Could you check a few things on this model? Use its own coordinates, in mm. A direction names the side the tool comes from. Give positions to 0.01 mm unless a question says otherwise; leave off trailing zeros. Loops run counter-clockwise (first coordinate to the right, second up) from the corner with the lowest first, then second, coordinate; pieces in that order, holes last. Notation, with made-up numbers: (71.25, 42.25) - (127.25, 42.25) arc R7 cw to (127.25, 48.25) - close; hole circle Ø6 at (22, -21.5). An arc over 180 degrees is marked (long way). Write each question's results on one line, items separated by ' | '. Start each with the question number.
1) I want a section at D-D, the plane y = 44. Write out the boundary of the cut face in (x, z) (3 decimals), and give its area (3 significant figures).
2) I'm going to push flat-ended pins straight in: pin 1 (2 mm diameter, centred on x = 0, z = -22, fed in from +Y); pin 2 (3 mm diameter, centred on x = 0, z = -189, fed in from +Y); pin 3 (1 mm diameter, centred on x = -0.5, y = 2.5, fed in from -Z). Where does each tip first touch, or does it pass through?
3) If we mould it in two halves opening along Y, with no side actions, what happens to faces 1 (the face through (0.044, -31.253, -213.834)), 2 (the face through (0, -21, -216.22)), 3 (the face through (0, -24.244, -107))? For each: +Y half, -Y half, draft (parallel to the pull), parting line (faces both ways), or undercut.
4) I want a section at B-B, the plane x = -1.5. Count the separate pieces of the cut face and the enclosed holes in it, and give its area (3 significant figures).
5) On a 3-axis mill with a long thin cutter (end or side, diameter ignored), from which of +Z, -Z, +X, -X, +Y, -Y can I reach the whole of each face in a straight line? I mean faces 4 (the face through (0, -33.769, -127)), 5 (the face through (0.044, 32.874, -211.617)), 6 (the face through (0.044, 0.201, -216.993)). Say none if no direction works.
6) I want a section at A-A, the plane z = 0. Write out the boundary of the cut face in (x, y) (3 decimals).
7) I want a section at C-C, the plane z = -102.5. Write out the boundary of the cut face in (x, y) (3 decimals).
8) If I drill on probe 1 along Y at (x, z) = (1.25, -196); probe 2 along Y at (x, z) = (0.5, -207); probe 3 along Y at (x, z) = (-0.25, -124.5), over which ranges is the centre line in solid material (lowest first)? Write a range as [from, to].
from build123d import *

# Parameters (mm, degrees)
SKETCH1_R           = 27.5
SKETCH1_R_2         = 3.175
BOSS_EXTRUDE1_DEPTH = 3.175


with BuildPart() as part:
    # Sketch1 → Boss-Extrude1 (new, symmetric)
    with BuildSketch(Plane(origin=(0, 0, 0), x_dir=(0, 0, -1), z_dir=(1, 0, 0))):
        with BuildLine():
            Line((43.290925291, 33.7693), (207.850950123, 33.7693))
            ThreePointArc((207.850950123, 33.7693), (211.66677379, 32.848803409), (214.643231519, 30.28979508))
            ThreePointArc((214.643231519, 30.28979508), (218.030702378, 27.377418378), (222.373445551, 26.329812242))
            Line((222.373445551, 26.329812242), (225.811462365, 26.329812242))
            ThreePointArc((225.811462365, 26.329812242), (234.009351835, 19.645680106), (229.112770692, 10.26983309))
            ThreePointArc((229.112770692, 10.26983309), (224.916562194, 6.758274432), (223.344950123, 1.517163342))
            Line((223.344950123, 1.517163342), (223.344950123, -4.239874171))
            ThreePointArc((223.344950123, -4.239874171), (222.587277992, -7.247924869), (220.495070123, -9.538143699))
            ThreePointArc((220.495070123, -9.538143699), (217.356758318, -12.973471943), (216.220250123, -17.48554799))
            Line((216.220250123, -17.48554799), (216.220250123, -25.4))
            ThreePointArc((216.220250123, -25.4), (213.768938906, -31.317988784), (207.850950123, -33.7693))
            Line((207.850950123, -33.7693), (43.290925291, -33.7693))
            ThreePointArc((43.290925291, -33.7693), (39.64603709, -34.49427642), (36.555995713, -36.558845406))
            ThreePointArc((36.555995713, -36.558845406), (-51.7, 0), (36.555995713, 36.558845406))
            ThreePointArc((36.555995713, 36.558845406), (39.64603709, 34.49427642), (43.290925291, 33.7693))
        make_face()
        Circle(SKETCH1_R, mode=Mode.SUBTRACT)
        with Locations((161.512193823, 25.4)):
            Circle(SKETCH1_R_2, mode=Mode.SUBTRACT)
        with Locations((161.512193823, -25.4)):
            Circle(SKETCH1_R_2, mode=Mode.SUBTRACT)
        with BuildLine():
            Line((75.9443, 24.2443), (137.267893823, 24.2443))
            ThreePointArc((137.267893823, 24.2443), (161.512193823, 0), (137.267893823, -24.2443))
            Line((137.267893823, -24.2443), (75.9443, -24.2443))
            ThreePointArc((75.9443, -24.2443), (51.7, 0), (75.9443, 24.2443))
        make_face(mode=Mode.SUBTRACT)
        with BuildLine():
            Line((182.450950123, 9.144), (207.850950123, 9.144))
            ThreePointArc((207.850950123, 9.144), (216.994950123, 0), (207.850950123, -9.144))
            Line((207.850950123, -9.144), (182.450950123, -9.144))
            ThreePointArc((182.450950123, -9.144), (173.306950123, 0), (182.450950123, 9.144))
        make_face(mode=Mode.SUBTRACT)
        with BuildLine():
            Line((164.490437881, -15.941212242), (189.890437881, -15.941212242))
            ThreePointArc((189.890437881, -15.941212242), (191.909737881, -17.960512242), (189.890437881, -19.979812242))
            Line((189.890437881, -19.979812242), (164.490437881, -19.979812242))
            ThreePointArc((164.490437881, -19.979812242), (162.471137881, -17.960512242), (164.490437881, -15.941212242))
        make_face(mode=Mode.SUBTRACT)
        with BuildLine():
            Line((200.411462365, 19.979812242), (225.811462365, 19.979812242))
            ThreePointArc((225.811462365, 19.979812242), (227.830762365, 17.960512242), (225.811462365, 15.941212242))
            Line((225.811462365, 15.941212242), (200.411462365, 15.941212242))
            ThreePointArc((200.411462365, 15.941212242), (198.392162365, 17.960512242), (200.411462365, 19.979812242))
        make_face(mode=Mode.SUBTRACT)
        with BuildLine():
            Line((182.450950123, 27.4193), (207.850950123, 27.4193))
            ThreePointArc((207.850950123, 27.4193), (209.870250123, 25.4), (207.850950123, 23.3807))
            Line((207.850950123, 23.3807), (182.450950123, 23.3807))
            ThreePointArc((182.450950123, 23.3807), (180.431650123, 25.4), (182.450950123, 27.4193))
        make_face(mode=Mode.SUBTRACT)
        with BuildLine():
            Line((182.450950123, -23.3807), (207.850950123, -23.3807))
            ThreePointArc((207.850950123, -23.3807), (209.870250123, -25.4), (207.850950123, -27.4193))
            Line((207.850950123, -27.4193), (182.450950123, -27.4193))
            ThreePointArc((182.450950123, -27.4193), (180.431650123, -25.4), (182.450950123, -23.3807))
        make_face(mode=Mode.SUBTRACT)
    extrude(amount=BOSS_EXTRUDE1_DEPTH, both=True)


solid = part.part
Answers:
1) outline: (-3.175, -27.146) - (3.175, -27.146) - (3.175, 27.146) - (-3.175, 27.146) - close | area: 345 mm2
2) pin 1: stops at y = 47.24 | pin 2: stops at y = 33.77 | pin 3: stops at z = -223.46
3) face 1: -Y half | face 2: draft | face 3: undercut
4) separate pieces: 1 | enclosed holes: 9 | area: 11,700 mm2
5) face 4: -Z, +X, -X, -Y | face 5: -Z, +X, -X, +Y | face 6: +X, -X
6) outline: (-3.175, -51.7) - (3.175, -51.7) - (3.175, -27.5) - (-3.175, -27.5) - close; (-3.175, 27.5) - (3.175, 27.5) - (3.175, 51.7) - (-3.175, 51.7) - close
7) outline: (-3.175, -33.769) - (3.175, -33.769) - (3.175, -24.244) - (-3.175, -24.244) - close; (-3.175, 24.244) - (3.175, 24.244) - (3.175, 33.769) - (-3.175, 33.769) - close
8) probe 1: y = [-33.77, -27.42], [-23.38, -9.14], [9.14, 23.38], [27.42, 33.77] | probe 2: y = [-33.77, -27.42], [-23.38, -9.14], [9.14, 15.94], [19.98, 23.38], [27.42, 33.77] | probe 3: y = [-33.77, -24.24], [24.24, 33.77]
